Work out the finished part from the listing and answer in its coordinate system (mm). Give positions to 0.01 mm unless a question says otherwise; leave off trailing zeros. Loops run counter-clockwise (first coordinate to the right, second up) from the corner with the lowest first, then second, coordinate; pieces in that order, holes last. Notation, with made-up numbers: (-13, 76) - (14, 76) arc R18 ccw to (14, 88) - close; hole circle Ø11 at (41.25, 52). An arc over 180 degrees is marked (long way). Use CSV: the item, a comma, the result in double quotes.
from build123d import *

# Parameters (mm, degrees)
F1_DEPTH = 12.7


with BuildPart() as f1:
    # F0 (on Front) → F1 (new body)
    with BuildSketch(Plane.XZ):
        with BuildLine():
            Line((0, 152.4), (0, 0))
            Line((0, 0), (101.6, 0))
            ThreePointArc((101.6, 0), (457.2, 37.801961), (812.8, 0))
            Line((812.8, 0), (914.4, 0))
            Line((914.4, 0), (914.4, 152.4))
            Line((914.4, 152.4), (0, 152.4))
        make_face()
    extrude(amount=-F1_DEPTH)


solid = f1.part
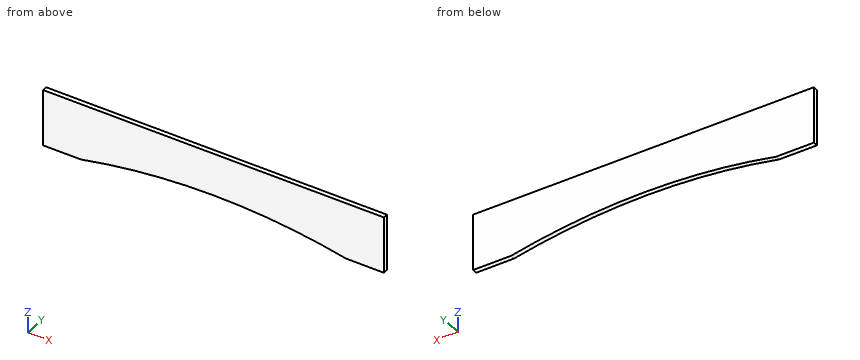
Item 1: A cutting plane is placed at A-A on z = 27. Determine the outline of the cut face in (x, y), and give its area (3 significant figures).
Determined:
outline,"(0, 0) - (266.35, 0) - (266.35, 12.7) - (0, 12.7) - close; (648.05, 0) - (914.4, 0) - (914.4, 12.7) - (648.05, 12.7) - close"
area,"6,770 mm²"
Item 2: A cutting plane is placed at D-D on x = 112.5. Determine the outline of the cut face in (y, z).
Determined:
outline,"(0, 2.31) - (12.7, 2.31) - (12.7, 152.4) - (0, 152.4) - close"
Item 3: A cutting plane is placed at C-C on x = 407. Determine the outline of the cut face in (y, z).
Determined:
outline,"(0, 37.06) - (12.7, 37.06) - (12.7, 152.4) - (0, 152.4) - close"
Item 4: A cutting plane is placed at B-B on y = 4. Determine the outline of the cut face in (x, z), and give its area (3 significant figures).
Determined:
outline,"(0, 0) - (101.6, 0) arc R1691.45 cw to (812.8, 0) - (914.4, 0) - (914.4, 152.4) - (0, 152.4) - close"
area,"121,000 mm²"
Item 5: Find the intervals of material crossed by line 1 (Z direction, x = 735.5, y = 8.75); line 2 (Z direction, x = 660, y = 7.5), in increasing order.
Determined:
line 1,"z = 14.75 to 152.4"
line 2,"z = 25.6 to 152.4"
